Geometry check sheet. Reference: the model listing, model coordinates, mm. A direction names the side the tool comes from. Give positions to 0.01 mm unless a question says otherwise; leave off trailing zeros. Loops run counter-clockwise (first coordinate to the right, second up) from the corner with the lowest first, then second, coordinate; pieces in that order, holes last. Notation, with made-up numbers: (35, 69.5) - (78, 69.5) arc R18 cw to (78, 103.5) - close; hole circle Ø10 at (4.25, 76.25). An arc over 180 degrees is marked (long way). Use a Markdown table: item, result. Add a question column.
1. Cross-section at A-A on z = -76.2. Enter the section's corners in (x, y), and give its area (3 significant figures).
2. Cross-section at B-B on y = -5.2. Enter the section's corners in (x, z).
3. Depth check by flat-ended pin: P1, Ø3, axis at x = 84, z = -78.5, coming from the +Y side; P2, Ø2, axis at y = -6.5, z = -78.5, coming from the +X side; P3, Ø1, axis at y = -5, z = -79, coming from the -X side. Enter the tip coordinate at first touch or a pass-through.
4. Draft check along Y on faces 1 (the cylindrical face through (89.29, -6.36, -78.72)), 2 (the cylindrical face through (89.85, -3.63, -75.99)), 3 (the flat face through (83.55, -5, -79)). Enter one of: pulls with the +Y half, pulls with the -Y half, needs draft (parallel to the pull), parting line crosses it, or undercut.
5. Material ranges on L1, parallel to Z at x = 83.5, y = -6.5; L2, parallel to X at y = -5.7, z = -77.55; L3, parallel to Y at x = 85.5, z = -79.2, recorded low to high.
6. Set-up check for faces 4 (the cylindrical face through (83.81, -4.2, -78.72)), 5 (the cylindrical face through (83.82, -6.37, -78.72)), 6 (the flat face through (89.55, -5, -79)), 7 (the flat face through (87, -6.63, -79)), 8 (the cylindrical face through (89, -4, -79)): record each of +Z, -Z, +X, -X, +Y, -Y from which the full face is reachable in a straight line by a thin tool's end or side.
from build123d import *

# Parameters (mm, degrees)
EXTRUDE230_DEPTH          = 1
EXTRUDE229_DEPTH          = 5
FUSION223_PLACEMENT_ANGLE = 90


with BuildPart() as extrude230:
    # Sketch232 → Extrude230 (new body)
    with BuildSketch(Plane.XZ):
        with BuildLine():
            ThreePointArc((11.7, 16.35), (11.063604, 16.086396), (10.8, 15.45))
            Line((10.8, 14.2), (10.8, 15.45))
            ThreePointArc((10.8, 14.2), (11.23934, 13.13934), (12.3, 12.7))
            Line((16.8, 12.7), (12.3, 12.7))
            ThreePointArc((16.8, 12.7), (17.86066, 13.13934), (18.3, 14.2))
            Line((18.3, 15.45), (18.3, 14.2))
            ThreePointArc((18.3, 15.45), (18.036396, 16.086396), (17.4, 16.35))
            Line((11.7, 16.35), (17.4, 16.35))
        make_face()
    extrude(amount=EXTRUDE230_DEPTH)


with BuildPart() as extrude230_1:
    # Extrude230 placement: moved
    add(extrude230.part.moved(Location((0, 2.5, 0))))


with BuildPart() as button005:
    # Sketch231 → Extrude229 (new body)
    with BuildSketch(Plane.XZ):
        with BuildLine():
            ThreePointArc((12.75, 16.23), (12.113604, 15.966396), (11.85, 15.33))
            Line((11.85, 14.43), (11.85, 15.33))
            ThreePointArc((11.85, 14.43), (12.113604, 13.793604), (12.75, 13.53))
            Line((16.95, 13.53), (12.75, 13.53))
            ThreePointArc((16.95, 13.53), (17.586396, 13.793604), (17.85, 14.43))
            Line((17.85, 15.33), (17.85, 14.43))
            ThreePointArc((17.85, 15.33), (17.586396, 15.966396), (16.95, 16.23))
            Line((12.75, 16.23), (16.95, 16.23))
        make_face()
    extrude(amount=EXTRUDE229_DEPTH)


with BuildPart() as button005_1:
    # Extrude229 placement: moved
    add(button005.part.moved(Location((-0.3, 2, -0.1))))

    # Fusion223: union Extrude230
    add(extrude230_1.part)


with BuildPart() as button005_2:
    # Fusion223 placement: moved
    add(button005_1.part.moved(Location((72, 9.5, -78))).rotate(Axis((72, 9.5, -78), (1, 0, 0)), FUSION223_PLACEMENT_ANGLE))


solid = button005_2.part
Values found:
| question | item | result |
|---|---|---|
| 1 | outline | (82.8, -5.95) arc R0.9 ccw to (83.7, -6.85) - (89.4, -6.85) arc R0.9 ccw to (90.3, -5.95) - (90.3, -4.7) arc R1.5 ccw to (88.8, -3.2) - (84.3, -3.2) arc R1.5 ccw to (82.8, -4.7) - close |
| 1 | area | 26.1 mm2 |
| 2 | outline | (82.8, -76.5) - (83.55, -76.5) - (83.55, -81) - (89.55, -81) - (89.55, -76.5) - (90.3, -76.5) - (90.3, -75.5) - (82.8, -75.5) - close |
| 3 | P1 | stops at y = -3.93 |
| 3 | P2 | stops at x = 89.55 |
| 3 | P3 | stops at x = 83.55 |
| 4 | face 1 | pulls with the -Y half |
| 4 | face 2 | pulls with the +Y half |
| 4 | face 3 | needs draft |
| 5 | L1 | z = -76.5 to -75.5 |
| 5 | L2 | x = 83.55 to 89.55 |
| 5 | L3 | y = -6.63 to -3.93 |
| 6 | face 4 | -Z, -X, +Y |
| 6 | face 5 | -Z, -X, -Y |
| 6 | face 6 | -Z, +X, +Y, -Y |
| 6 | face 7 | -Z, +X, -X, -Y |
| 6 | face 8 | -Z, +X, +Y |
